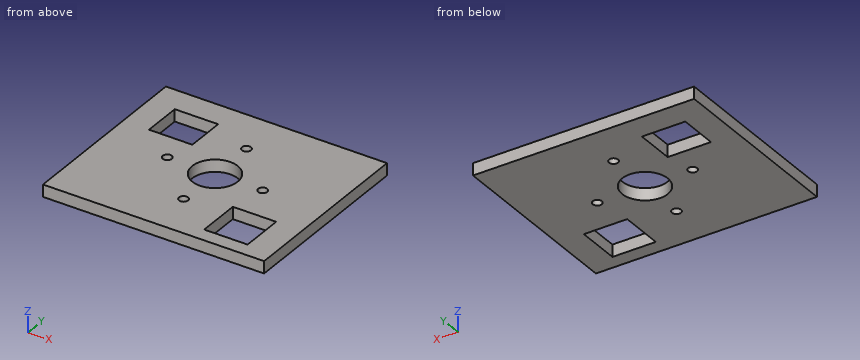
from build123d import *

# Parameters (mm, degrees)
F0_W     = 51
F0_H     = 43
F0_R     = 1.05
F0_W_2   = 10
F0_H_2   = 10
F0_R_2   = 5.25
F0_H_3   = 9
F1_DEPTH = 2.8


with BuildPart() as f1:
    # F0 (on Top) → F1 (new body)
    with BuildSketch(Plane.XY):
        with Locations((-36.876488, 29.491607)):
            Rectangle(F0_W, F0_H)
        with Locations((-47.876488, 29.491607)):
            Circle(F0_R, mode=Mode.SUBTRACT)
        with Locations((-36.876488, 18.491607)):
            Circle(F0_R, mode=Mode.SUBTRACT)
        with Locations((-22.376488, 16.304032)):
            Rectangle(F0_W_2, F0_H_2, mode=Mode.SUBTRACT)
        with Locations((-36.876488, 29.491607)):
            Circle(F0_R_2, mode=Mode.SUBTRACT)
        with Locations((-25.876488, 29.491607)):
            Circle(F0_R, mode=Mode.SUBTRACT)
        with Locations((-51.376488, 40.491607)):
            Rectangle(F0_W_2, F0_H_3, mode=Mode.SUBTRACT)
        with Locations((-36.876488, 40.491607)):
            Circle(F0_R, mode=Mode.SUBTRACT)
    extrude(amount=F1_DEPTH)


solid = f1.part
Verification items for the finished model (mm, model axes). Round coordinates to 2 decimals unless told otherwise and drop trailing zeros. Write each loop counter-clockwise with the first axis right and the second up, starting at its lowest first coordinate (ties: lowest second). Pieces come first, ordered by that corner, then holes.
(1) Section check A-A (y = 25.5). Enter the section's corners in (x, z), plus the area to 3 significant figures.
Returned:
outline: (-62.38, 0) - (-40.29, 0) - (-40.29, 2.8) - (-62.38, 2.8) - close; (-33.47, 0) - (-11.38, 0) - (-11.38, 2.8) - (-33.47, 2.8) - close
area: 124 mm2
(2) Depth check by flat-ended pin: pin 1 Ø1.3 at (x, y) = (-25.88, 29.49) entering from +Z. Enter the tip coordinate at first touch or a pass-through.
Returned:
pin 1: passes through
(3) Material ranges on line 1 (Y direction, x = -23, z = 0.8); line 2 (X direction, y = 37.5, z = 2.4); line 3 (X direction, y = 30, z = 0.6), recorded low to high.
Returned:
line 1: y = 7.99 to 11.3, 21.3 to 50.99
line 2: x = -62.38 to -56.38, -46.38 to -11.38
line 3: x = -62.38 to -48.8, -46.96 to -42.1, -31.65 to -26.8, -24.96 to -11.38
(4) Section check B-B (z = 1.4). Enter the section's corners in (x, y).
Returned:
outline: (-62.38, 7.99) - (-11.38, 7.99) - (-11.38, 50.99) - (-62.38, 50.99) - close; hole (-56.38, 35.99) - (-46.38, 35.99) - (-46.38, 44.99) - (-56.38, 44.99) - close; hole circle Ø2.1 at (-47.88, 29.49); hole circle Ø10.5 at (-36.88, 29.49); hole circle Ø2.1 at (-36.88, 18.49); hole circle Ø2.1 at (-36.88, 40.49); hole (-27.38, 11.3) - (-17.38, 11.3) - (-17.38, 21.3) - (-27.38, 21.3) - close; hole circle Ø2.1 at (-25.88, 29.49)
(5) Section check C-C (y = 20.5). Enter the section's corners in (x, z).
Returned:
outline: (-62.38, 0) - (-27.38, 0) - (-27.38, 2.8) - (-62.38, 2.8) - close; (-17.38, 0) - (-11.38, 0) - (-11.38, 2.8) - (-17.38, 2.8) - close
